Verification items for the finished model (mm, model axes). Give positions to 0.01 mm unless a question says otherwise; leave off trailing zeros. Loops run counter-clockwise (first coordinate to the right, second up) from the corner with the lowest first, then second, coordinate; pieces in that order, holes last. Notation, with made-up numbers: M 29,70 L 83,70 A22 ccw 83,109 Z; hole C -40,18 d1. An arc over 180 degrees is marked long. Answer in a Markdown table with one row per item.
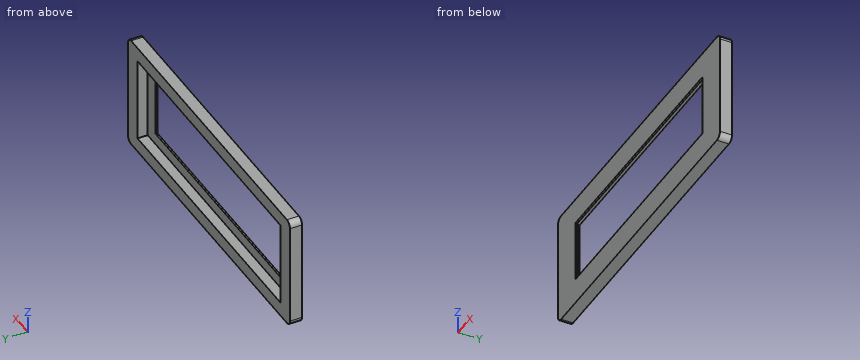
```python
from build123d import *

# Parameters (mm, degrees)
F0_W     = 103.410944
F0_H     = 37.954018
F0_W_2   = 81.041918
F0_H_2   = 20.718862
F1_DEPTH = 4
F2_W     = 91.309666
F2_H     = 28.419676
F2_W_2   = 81.041918
F2_H_2   = 20.718862
F3_DEPTH = 3.4
F4_R     = 2


with BuildPart() as f1:
    # F0 (on Front) → F1 (new body)
    with BuildSketch(Plane.XZ):
        Rectangle(F0_W, F0_H)
        Rectangle(F0_W_2, F0_H_2, mode=Mode.SUBTRACT)
    extrude(amount=F1_DEPTH)

    # F2 (on face) → F3 (cut)
    with BuildSketch(Plane(origin=(0, 0, 0), x_dir=(-1, 0, 0), z_dir=(0, 1, 0))):
        Rectangle(F2_W, F2_H)
        Rectangle(F2_W_2, F2_H_2, mode=Mode.SUBTRACT)
    extrude(amount=-F3_DEPTH, mode=Mode.SUBTRACT)

    # F4
    f4_edges = [f1.edges().sort_by_distance(p)[0] for p in [
        (-51.705472, -2, 18.977009),
        (51.705472, -2, 18.977009),
        (51.705472, -2, -18.977009),
        (-51.705472, -2, -18.977009),
    ]]
    fillet(f4_edges, radius=F4_R)


solid = f1.part
```
Item 1: Sectioned sample at C-C (z = 8). Record the cut outline in (x, y), and give its area (3 significant figures).
Reported:
| item | result |
|---|---|
| outline | M -51.71,-4 L -40.52,-4 L -40.52,-3.4 L -45.65,-3.4 L -45.65,0 L -51.71,0 Z; M 40.52,-4 L 51.71,-4 L 51.71,0 L 45.65,0 L 45.65,-3.4 L 40.52,-3.4 Z |
| area | 54.6 mm^2 |
Item 2: Sectioned sample at B-B (y = -1.95). Record the cut outline in (x, z).
Reported:
| item | result |
|---|---|
| outline | M -51.71,-16.98 A2 ccw -49.71,-18.98 L 49.71,-18.98 A2 ccw 51.71,-16.98 L 51.71,16.98 A2 ccw 49.71,18.98 L -49.71,18.98 A2 ccw -51.71,16.98 Z; hole M -45.65,-14.21 L 45.65,-14.21 L 45.65,14.21 L -45.65,14.21 Z |
Item 3: Go/stop test with a flat-tipped pin: pin 1 (10 mm diameter, centred on x = -30, z = -14, fed in from +Y). Record where the tip stops, or that it passes through.
Reported:
| item | result |
|---|---|
| pin 1 | stops at y = 0 |
Item 4: Sectioned sample at D-D (z = -12.5). Record the cut outline in (x, y), and give its area (3 significant figures).
Reported:
| item | result |
|---|---|
| outline | M -51.71,-4 L 51.71,-4 L 51.71,0 L 45.65,0 L 45.65,-3.4 L -45.65,-3.4 L -45.65,0 L -51.71,0 Z |
| area | 103 mm^2 |
Item 5: Scan lines: L1, parallel to X at y = -2.8, z = 0; L2, parallel to Z at x = 16.5, y = -3.55; L3, parallel to Z at x = -29, y = -2.75. Record each from-to range of solid material in increasing order. Write a range as [from, to].
Reported:
| item | result |
|---|---|
| L1 | x = [-51.71, -45.65], [45.65, 51.71] |
| L2 | z = [-18.98, -10.36], [10.36, 18.98] |
| L3 | z = [-18.98, -14.21], [14.21, 18.98] |
Item 6: Sectioned sample at A-A (x = -23). Record the cut outline in (y, z), and give its area (3 significant figures).
Reported:
| item | result |
|---|---|
| outline | M -4,-18.98 L 0,-18.98 L 0,-14.21 L -3.4,-14.21 L -3.4,-10.36 L -4,-10.36 Z; M -4,10.36 L -3.4,10.36 L -3.4,14.21 L 0,14.21 L 0,18.98 L -4,18.98 Z |
| area | 42.8 mm^2 |
